Here's how the part is built. I have some questions about the finished solid (model axes, mm). Face numbers are marked on the shaded views. A direction names the side the tool comes from. Give positions to 0.01 mm unless a question says otherwise; leave off trailing zeros. Order: outer loops, then holes, each group sorted by start corner. A loop starts at its lowest first (then second) coordinate and runs counter-clockwise, first axis right, second up. Notation, with made-up numbers: M 64,-22 L 92,-22 A14 cw 92,5 Z; hole C 84.5,86.25 d10. An arc over 180 degrees is marked long. Use one line per item in the form item = value.
from build123d import *

# Parameters (mm, degrees)
F0_R            = 9.4221007419
F1_DEPTH        = 5.08
F3_DEPTH        = 5.08
F3_COPIES_COUNT = 19


# Not quite as in the source:
# - a pattern or mirror of a feature is missing from the dataset's text; its kind, count and spacing are read off the source's solid
# - a feature names something its author has since deleted; it is built from what else it names


with BuildPart() as f1:
    # F0 (on Top) → F1 (new body)
    with BuildSketch(Plane.XY):
        Circle(F0_R)
        with BuildLine():
            ThreePointArc((-2.6457529, -2.9999985987), (0, 4), (2.6457529, -2.9999985987))
            Line((2.6457529, -2.9999985987), (-2.6457529, -2.9999985987))
        make_face(mode=Mode.SUBTRACT)
    extrude(amount=F1_DEPTH)

    # F2 (on face) → F3 (cut, through all)
    with BuildSketch(Plane.XY.offset(5.08)):
        with BuildLine():
            Line((0.2702110818, 7.4907975301), (1.1292079793, 9.3541900628))
            ThreePointArc((1.1292079793, 9.3541900628), (0, 9.4221007419), (-1.1292079793, 9.3541900628))
            Line((-1.1292079793, 9.3541900628), (-0.2702110818, 7.4907975301))
            ThreePointArc((-0.2702110818, 7.4907975301), (0, 7.3178208914), (0.2702110818, 7.4907975301))
        make_face()
    f3 = extrude(amount=-F3_DEPTH, mode=Mode.SUBTRACT)

    # F3_copies: F3 ×19 about axis
    f3_copies_axis = Axis((0, 0, 0), (0, 0, 1))
    for i in range(1, F3_COPIES_COUNT):
        add(f3.rotate(f3_copies_axis, i * 360 / F3_COPIES_COUNT), mode=Mode.SUBTRACT)


solid = f1.part
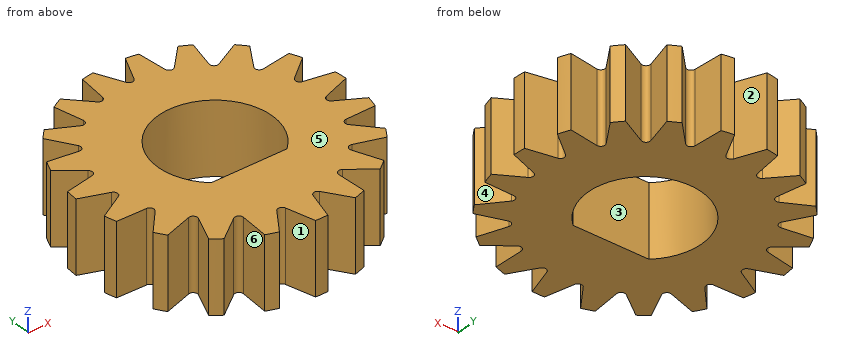
Q1. I need wall thicknesses on L1, parallel to Y at x = 7.25, z = 2.1; L2, parallel to Y at x = -7.5, z = 3.25; L3, parallel to Y at x = -8, z = 3.65. Which ranges of each line are inside material? Lowest first, please.
Found:
L1 = -5.38 to -3.82, -2.76 to 1.6, 2.15 to 3.99
L2 = -5.46 to -4.1, -2.75 to -0.92, -0.34 to 1.54, 2.35 to 4.03
L3 = -4.98 to -4.66, -2.74 to -1.2, -0.16 to 1.45, 2.75 to 4.1
Q2. Thinking about a two-plate mould opening in X: for the marked faces 4, 5 and 6, which applies, +X half, -X half, draft (parallel to the pull), parting line (faces both ways), or undercut?
Found:
face_4 = +X half
face_5 = draft
face_6 = undercut
Q3. I want a section at A-A on x = 0. Write out the boundary of the cut face in (y, z).
Found:
outline = M -9.42,0 L -3,0 L -3,5.08 L -9.42,5.08 Z; M 4,0 L 7.32,0 L 7.32,5.08 L 4,5.08 Z
Q4. I want a section at B-B on y = 0. Write out the boundary of the cut face in (x, z), then the cut area to 3 significant figures.
Found:
outline = M -8.45,0 L -4,0 L -4,5.08 L -8.45,5.08 Z; M 4,0 L 8.45,0 L 8.45,5.08 L 4,5.08 Z
area = 45.2 mm²
Q5. I'm going to push a flat-ended pin straight in: pin 1 Ø3 at (x, z) = (-2.5, 4) entering from -Y. Where does the tip first touch, or does it pass through?
Found:
pin_1 = -9.04
Q6. I want a section at C-C on y = -6. Write out the boundary of the cut face in (x, z), then the cut area to 3 significant figures.
Found:
outline = M -5.63,0 L 5.63,0 L 5.63,5.08 L -5.63,5.08 Z
area = 57.2 mm²
Q7. On a 3-axis mill with a long thin cutter (end or side, diameter ignored), from which of +Z, -Z, +X, -X, +Y, -Y can I reach the whole of each face in a straight line? I mean the marked faces 1, 2 and 3. Say none if no direction works.
Found:
face_1 = +Z, -Z, -Y
face_2 = +Z, -Z, +Y
face_3 = +Z, -Z
